Drawing for the job (mm, zero at the part's lowest x, y, z). A direction names the side the tool comes from. Give positions to 0.01 mm unless a question says otherwise; leave off trailing zeros. Loops run counter-clockwise (first coordinate to the right, second up) from the corner with the lowest first, then second, coordinate; pieces in that order, holes last. Notation, with made-up numbers: M -15,0 L 20,0 A33 cw 20,29 Z; hole C 70.25,-36 d5. An arc over 180 degrees is marked long. Answer in a Markdown table with one row per item. Add a question column.
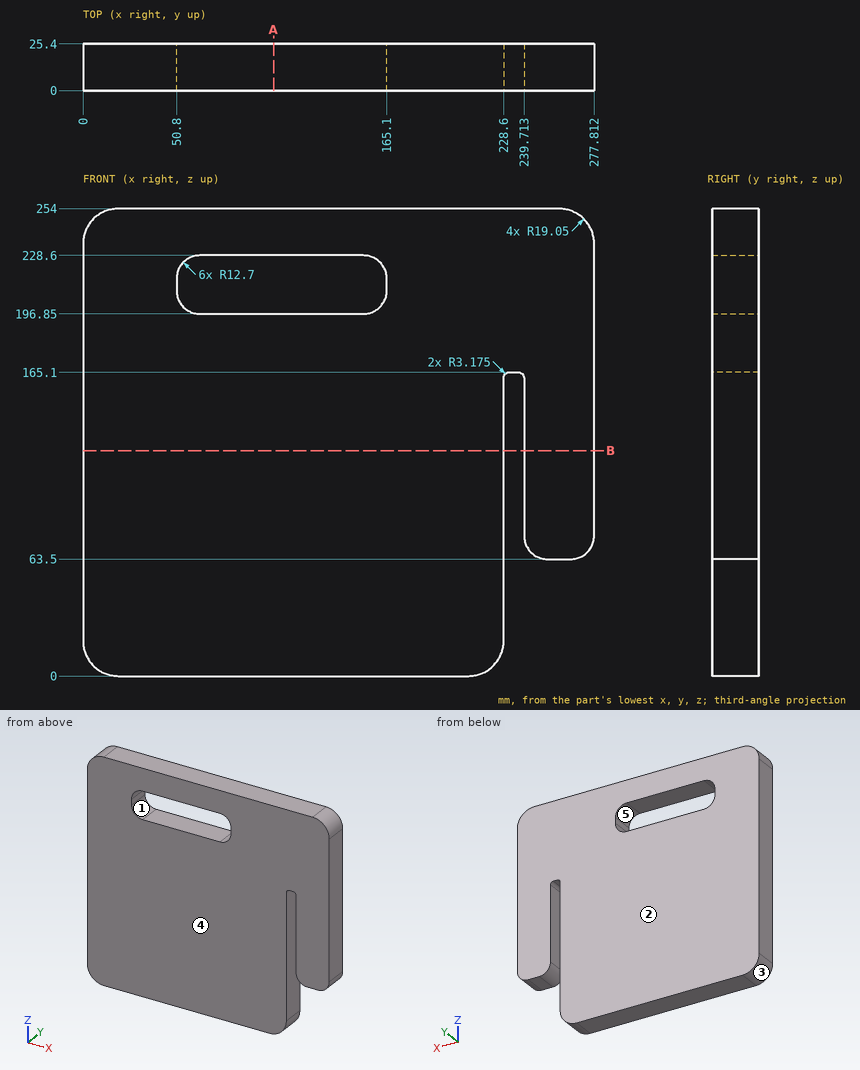
(1) Slice it at B-B, the plane z = 122.5. Give the cut face in (x, y).
(2) Pull direction Z, two halves, no side cores. Call the marked faces 3, 4 and 5: +Z half, -Z half, draft (parallel to the pull), parting line (faces both ways), or undercut.
(3) Wall check: line 1 (Z direction, x = 77, y = 23); line 2 (X direction, y = 13.5, z = 112.5); line 3 (X direction, y = 9.25, z = 209). Give the ranges that are in metal, low to high.
(4) Tool access for the marked faces 1 and 2: list every direction of +Z, -Z, +X, -X, +Y, -Y with a clear straight run to the whole face (end or side of a thin tool).
(5) Pin check, flat tips, straight feed: pin 1 (5 mm diameter, centred on x = 234, y = 12.5, fed in from -Z); pin 2 (10 mm diameter, centred on x = 259, y = 14, fed in from -Z). Stop position of each tip, or through.
(6) Slice it at A-A, the plane x = 103.5. Give the cut face in (y, z).
Solution:
| question | item | result |
|---|---|---|
| 1 | outline | M 0,0 L 228.6,0 L 228.6,25.4 L 0,25.4 Z; M 239.71,0 L 277.81,0 L 277.81,25.4 L 239.71,25.4 Z |
| 2 | face 3 | -Z half |
| 2 | face 4 | draft |
| 2 | face 5 | undercut |
| 3 | line 1 | 0 to 196.85, 228.6 to 254 |
| 3 | line 2 | 0 to 228.6, 239.71 to 277.81 |
| 3 | line 3 | 0 to 50.81, 165.09 to 277.81 |
| 4 | face 1 | +Y, -Y |
| 4 | face 2 | +Z, -Z, +X, -X, +Y |
| 5 | pin 1 | z = 165.09 |
| 5 | pin 2 | z = 63.5 |
| 6 | outline | M 0,0 L 25.4,0 L 25.4,196.85 L 0,196.85 Z; M 0,228.6 L 25.4,228.6 L 25.4,254 L 0,254 Z |
